Source: CAD feature listing. Evaluate the final solid. Frame: model axes, mm. A direction names the side the tool comes from. Give positions to 0.01 mm unless a question says otherwise; leave off trailing zeros. Loops run counter-clockwise (first coordinate to the right, second up) from the corner with the lowest first, then second, coordinate; pieces in that order, holes last.
from build123d import *

# Parameters (mm, degrees)
SKETCH_1_R          = 1.75
EXTRUDE_1_DEPTH     = 3
SKETCH_2_R          = 12
EXTRUDE_2_DEPTH     = 2
SKETCH_3_R          = 4.5
SKETCH_3_R_2        = 3
EXTRUDE_3_DEPTH     = 3
SKETCH_4_R          = 3
CUT_EXTRUDE_1_DEPTH = 2
SKETCH_5_R          = 1.75
CUT_EXTRUDE_2_DEPTH = 9


with BuildPart() as part:
    # Эскиз1 → Бобышка-Вытянуть1 (new body)
    with BuildSketch(Plane(origin=(0, 0, 0), x_dir=(1, 0, 0), z_dir=(0, 1, 0))):
        with BuildLine():
            Line((-30, 5), (-11.456439237, 5))
            ThreePointArc((-11.456439237, 5), (-10.2750901, 7.118463559), (-8.706840344, 8.968886844))
            ThreePointArc((-8.706840344, 8.968886844), (-8.255178852, 9.942485712), (-8.569645055, 10.968645479))
            Line((-8.569645055, 10.968645479), (-8.619260655, 11.03215055))
            ThreePointArc((-8.619260655, 11.03215055), (8.619260655, 11.03215055), (12.789636407, -5.694313003))
            Line((12.789636407, -5.694313003), (12.716014607, -5.661534466))
            ThreePointArc((12.716014607, -5.661534466), (11.644259912, -5.604659769), (10.808847895, -6.278439868))
            ThreePointArc((10.808847895, -6.278439868), (-0.716551297, -12.47944527), (-11.456439237, -5))
            Line((-11.456439237, -5), (-30, -5))
            ThreePointArc((-30, -5), (-35, 0), (-30, 5))
        make_face()
        with Locations((-30, 0)):
            Circle(SKETCH_1_R, mode=Mode.SUBTRACT)
    extrude(amount=EXTRUDE_1_DEPTH)

    # Эскиз2 → Бобышка-Вытянуть2 (add)
    with BuildSketch(Plane(origin=(0, 3, 0), x_dir=(1, 0, 0), z_dir=(0, 1, 0))):
        Circle(SKETCH_2_R)
    extrude(amount=EXTRUDE_2_DEPTH)

    # Эскиз3 → Бобышка-Вытянуть3 (add)
    with BuildSketch(Plane(origin=(0, 5, 0), x_dir=(1, 0, 0), z_dir=(0, 1, 0))):
        Circle(SKETCH_3_R)
        Circle(SKETCH_3_R_2, mode=Mode.SUBTRACT)
    extrude(amount=EXTRUDE_3_DEPTH)

    # Эскиз4 → Вырез-Вытянуть1 (cut)
    with BuildSketch(Plane(origin=(0, 5, 0), x_dir=(1, 0, 0), z_dir=(0, 1, 0))):
        Circle(SKETCH_4_R)
    extrude(amount=-CUT_EXTRUDE_1_DEPTH, mode=Mode.SUBTRACT)

    # Эскиз5 → Вырез-Вытянуть2 (cut, through all)
    with BuildSketch(Plane(origin=(0, 8, 0), x_dir=(1, 0, 0), z_dir=(0, 1, 0))):
        Circle(SKETCH_5_R)
        with Locations((-7, 0)):
            Circle(SKETCH_5_R)
        with Locations((7, 0)):
            Circle(SKETCH_5_R)
    extrude(amount=-CUT_EXTRUDE_2_DEPTH, mode=Mode.SUBTRACT)


solid = part.part
1) Cut plane D-D (y = 7.5). Return loops of the section in (x, z), and give its area (3 significant figures).
Checks:
outline: circle Ø9 at (0, 0); hole circle Ø6 at (0, 0)
area: 35.3 mm2
2) Contact query for flat-ended pins moving along their axis: P1, Ø7, axis at x = 0, z = 0, coming from the -Y side; P2, Ø0.9, axis at x = -19.5, y = 1, coming from the +Z side; P3, Ø1, axis at x = -23, z = 6, coming from the +Y side; P4, Ø4, axis at x = -30, z = 0, coming from the +Y side. Output: stop coordinate, or through.
Checks:
P1: stops at y = 0
P2: stops at z = 5
P3: passes through
P4: stops at y = 3
3) Cut plane A-A (z = 0). State how many separate pieces and enclosed holes the cut face has, and give its area (3 significant figures).
Checks:
separate pieces: 5
enclosed holes: 0
area: 136 mm2
4) Cut plane B-B (x = 7). Return loops of the section in (y, z).
Checks:
outline: (0, -12.12) - (3, -12.12) - (3, -9.75) - (5, -9.75) - (5, -1.75) - (0, -1.75) - close; (0, 1.75) - (5, 1.75) - (5, 9.75) - (3, 9.75) - (3, 10.36) - (0, 10.36) - close
5) Cut plane C-C (y = 1). Return loops of the section in (x, z).
Checks:
outline: (-30, -5) - (-11.46, -5) arc R12.5 ccw to (-8.71, -8.97) arc R1.5 cw to (-8.57, -10.97) - (-8.62, -11.03) arc R14 ccw to (12.79, 5.69) - (12.72, 5.66) arc R1.5 cw to (10.81, 6.28) arc R12.5 ccw to (-11.46, 5) - (-30, 5) arc R5 ccw to start; hole circle Ø3.5 at (-30, 0); hole circle Ø3.5 at (-7, 0); hole circle Ø3.5 at (0, 0); hole circle Ø3.5 at (7, 0)
6) Pull-direction query (X, two-part tool) for faces 1 (the cylindrical face through (-0.59, 6.48, -4.46)), 2 (the cylindrical face through (1.617, 1.521, 0.67)), 3 (the cylindrical face through (-8.256, 1.479, -9.927)); classes: released by +X, released by -X, zero draft, split by the parting line, or undercut.
Checks:
face 1: split by the parting line
face 2: undercut
face 3: released by -X
7) Reachability of faces 4 (the flat face through (-5, 0, -1)), 5 (the flat face through (-21, 1, -5)), 6 (the flat face through (-21, 1, 5)), 7 (the cylindrical face through (-11.99, 3.99, -0.53)) from +Z, -Z, +X, -X, +Y, -Y: full face, straight path, thin tool, end or side. Return the list, or none.
Checks:
face 4: +Z, -Z, +X, -X, -Y
face 5: -Z, -X, +Y, -Y
face 6: +Z, -X, +Y, -Y
face 7: +Y
8) Ray query, probe 1 along X at (y, z) = (4.5, 0); probe 2 along X at (y, z) = (2.65, 0); probe 3 along X at (y, z) = (6, 0). Return the intervals inside material, ascending.
Checks:
probe 1: x = -12 to -8.75, -5.25 to -3, 3 to 5.25, 8.75 to 12
probe 2: x = -35 to -31.75, -28.25 to -8.75, -5.25 to -1.75, 1.75 to 5.25, 8.75 to 14
probe 3: x = -4.5 to -3, 3 to 4.5
